```python
from build123d import *

# Parameters (mm, degrees)
SKETCH1_W               = 673.1
SKETCH1_H               = 444.5
BOSS_EXTRUDE1_DEPTH     = 0.1016
SKETCH2_W               = 569.9252
SKETCH2_H               = 309.5752
CUT_EXTRUDE1_DEPTH      = 1
CUT_EXTRUDE1_DEPTH_BACK = 1.2032


with BuildPart() as part:
    # Sketch1 → Boss-Extrude1 (new body, symmetric)
    with BuildSketch(Plane.XY):
        Rectangle(SKETCH1_W, SKETCH1_H)
    extrude(amount=BOSS_EXTRUDE1_DEPTH, both=True)

    # Sketch2 → Cut-Extrude1 (cut, two sides)
    with BuildSketch(Plane.XY.offset(0.1016)) as cut_extrude1_sk:
        Rectangle(SKETCH2_W, SKETCH2_H)
    extrude(amount=CUT_EXTRUDE1_DEPTH, mode=Mode.SUBTRACT)
    extrude(cut_extrude1_sk.sketch, amount=-CUT_EXTRUDE1_DEPTH_BACK, mode=Mode.SUBTRACT)


solid = part.part
```
Geometry: final body of the model. Coordinates: model frame, mm. Round coordinates to 2 decimals unless told otherwise and drop trailing zeros. Write each loop counter-clockwise with the first axis right and the second up, starting at its lowest first coordinate (ties: lowest second). Pieces come first, ordered by that corner, then holes. Notation, with made-up numbers: (84.25, -3) -> (105.25, -3) arc R32 ccw to (105.25, 23) -> close; hole circle Ø4 at (-23.75, 82). An arc over 180 degrees is marked (long way). Return JSON: item names as keys, results as strings.
Q1. Ray query, line 1 (X direction, y = -98, z = 0); line 2 (Y direction, x = 114, z = 0.05). Return the intervals inside material, ascending.
From the geometry:
{"line 1": "-336.55 to -284.96, 284.96 to 336.55", "line 2": "-222.25 to -154.79, 154.79 to 222.25"}
Q2. Section C-C on y = 47. Return the cut outline in (x, z).
From the geometry:
{"outline": "(-336.55, -0.1) -> (-284.96, -0.1) -> (-284.96, 0.1) -> (-336.55, 0.1) -> close; (284.96, -0.1) -> (336.55, -0.1) -> (336.55, 0.1) -> (284.96, 0.1) -> close"}
Q3. Section B-B on z = 0.05. Return the cut outline in (x, y), and give its area (3 significant figures).
From the geometry:
{"outline": "(-336.55, -222.25) -> (336.55, -222.25) -> (336.55, 222.25) -> (-336.55, 222.25) -> close; hole (-284.96, -154.79) -> (284.96, -154.79) -> (284.96, 154.79) -> (-284.96, 154.79) -> close", "area": "123,000 mm2"}
Q4. Section A-A on x = 57. Return the cut outline in (y, z), and give its area (3 significant figures).
From the geometry:
{"outline": "(-222.25, -0.1) -> (-154.79, -0.1) -> (-154.79, 0.1) -> (-222.25, 0.1) -> close; (154.79, -0.1) -> (222.25, -0.1) -> (222.25, 0.1) -> (154.79, 0.1) -> close", "area": "27.4 mm2"}
